from build123d import *

# Parameters (mm, degrees)
SKETCH_W      = 50.4
SKETCH_H      = 43.3
PAD_DEPTH     = 1.6
SKETCH001_R   = 1.65
HOLE_DEPTH    = 1.601
SKETCH002_W   = 10
SKETCH002_H   = 5.6
SKETCH002_W_2 = 5.6
SKETCH002_H_2 = 10
SKETCH002_W_3 = 5.7
SKETCH002_H_3 = 7.6
SKETCH002_W_4 = 7.6
SKETCH002_H_4 = 5.7
SKETCH002_H_5 = 9.8
PAD001_DEPTH  = 10.3


with BuildPart() as part:
    # Sketch → Pad (new body)
    with BuildSketch(Plane.XY):
        Rectangle(SKETCH_W, SKETCH_H)
    extrude(amount=PAD_DEPTH)

    # Sketch001 (on Face6 of Pad) → Hole (cut, through all)
    with BuildSketch(Plane.XY.offset(1.6)):
        with Locations((-22, 18.45)):
            Circle(SKETCH001_R)
        with Locations((22, 18.45)):
            Circle(SKETCH001_R)
        with Locations((-22, -18.45)):
            Circle(SKETCH001_R)
        with Locations((22, -18.45)):
            Circle(SKETCH001_R)
    extrude(amount=-HOLE_DEPTH, mode=Mode.SUBTRACT)

    # Sketch002 (on Face5 of Hole) → Pad001 (join)
    with BuildSketch(Plane.XY.offset(1.6)):
        with Locations((9.4, -17.35)):
            Rectangle(SKETCH002_W, SKETCH002_H)
        with Locations((-3.6, -17.35)):
            Rectangle(SKETCH002_W, SKETCH002_H)
        with Locations((-15.2, -14.25)):
            Rectangle(SKETCH002_W_2, SKETCH002_H_2)
        with Locations((-16.25, 9.05)):
            Rectangle(SKETCH002_W_3, SKETCH002_H_3)
        with Locations((5.2, 17.7)):
            Rectangle(SKETCH002_W_4, SKETCH002_H_4)
        with Locations((17.8, -8.15)):
            Rectangle(SKETCH002_W_4, SKETCH002_H_5)
    extrude(amount=PAD001_DEPTH)


solid = part.part
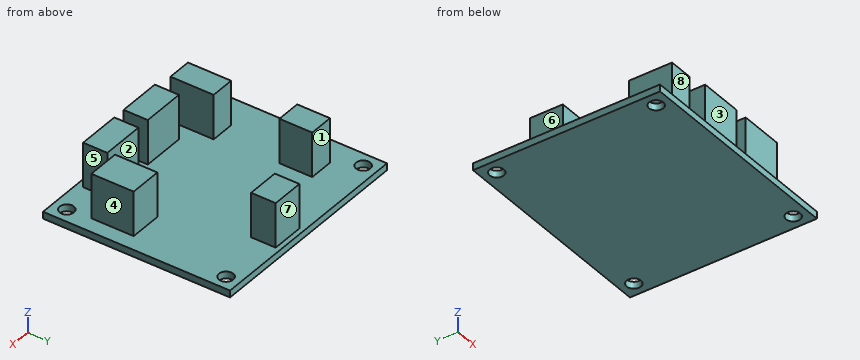
Work out the finished part from the listing and answer in its coordinate system (mm). Face numbers are marked on the shaded views. A direction names the side the tool comes from. Give positions to 0.01 mm unless a question says otherwise; leave off trailing zeros. Order: outer loops, then holes, each group sorted by start corner. A loop starts at its lowest first (then second) coordinate and runs counter-clockwise, first axis right, second up. Notation, with made-up numbers: M -5,-3.5 L 36,-3.5 A3 ccw 36,0.5 Z; hole C -13.5,-13 d6. An arc over 180 degrees is marked long. Return JSON: item names as keys, results as strings.
Q1. Find the intervals of material crossed by line 1 along X through (y, z) = (-15.5, 9); line 2 along Y through (x, z) = (-22, 0.75); line 3 along Z through (x, y) = (7, -6.5), in increasing order. Write a range as [from, to].
Answer below:
{"line 1": "x = [-18, -12.4], [-8.6, 1.4], [4.4, 14.4]", "line 2": "y = [-21.65, -20.1], [-16.8, 16.8], [20.1, 21.65]", "line 3": "z = [0, 1.6]"}
Q2. Find section B-B, the plane z = 4.5. Write down the section's boundary in (x, y).
Answer below:
{"outline": "M -19.1,5.25 L -13.4,5.25 L -13.4,12.85 L -19.1,12.85 Z; M -18,-19.25 L -12.4,-19.25 L -12.4,-9.25 L -18,-9.25 Z; M -8.6,-20.15 L 1.4,-20.15 L 1.4,-14.55 L -8.6,-14.55 Z; M 1.4,14.85 L 9,14.85 L 9,20.55 L 1.4,20.55 Z; M 4.4,-20.15 L 14.4,-20.15 L 14.4,-14.55 L 4.4,-14.55 Z; M 14,-13.05 L 21.6,-13.05 L 21.6,-3.25 L 14,-3.25 Z"}
Q3. Find section D-D, the plane x = -22. Write down the section's boundary in (y, z).
Answer below:
{"outline": "M -21.65,0 L -20.1,0 L -20.1,1.6 L -21.65,1.6 Z; M -16.8,0 L 16.8,0 L 16.8,1.6 L -16.8,1.6 Z; M 20.1,0 L 21.65,0 L 21.65,1.6 L 20.1,1.6 Z"}
Q4. Which of the six approach directions +Z, -Z, +X, -X, +Y, -Y give full straight-line access (tool end or side, diameter ignored) to the marked faces 5, 6, 7 and 8?
Answer below:
{"face 5": "+Z, +X, -Y", "face 6": "+Z, -X, +Y, -Y", "face 7": "+Z, +X, -X, +Y", "face 8": "+Z, -X, -Y"}
Q5. Find section A-A, the plane y = 18.45. Write down the section's boundary in (x, z).
Answer below:
{"outline": "M -25.2,0 L -23.65,0 L -23.65,1.6 L -25.2,1.6 Z; M -20.35,0 L 20.35,0 L 20.35,1.6 L 9,1.6 L 9,11.9 L 1.4,11.9 L 1.4,1.6 L -20.35,1.6 Z; M 23.65,0 L 25.2,0 L 25.2,1.6 L 23.65,1.6 Z"}
Q6. The mould has two halves that part along Y. Classify the marked faces 1, 2, 3 and 4: pulls with the +Y half, pulls with the -Y half, needs draft (parallel to the pull), parting line crosses it, or undercut.
Answer below:
{"face 1": "pulls with the +Y half", "face 2": "undercut", "face 3": "pulls with the -Y half", "face 4": "needs draft"}
Q7. Find section C-C, the plane x = 5. Write down the section's boundary in (y, z), and give its area (3 significant figures).
Answer below:
{"outline": "M -21.65,0 L 21.65,0 L 21.65,1.6 L 20.55,1.6 L 20.55,11.9 L 14.85,11.9 L 14.85,1.6 L -14.55,1.6 L -14.55,11.9 L -20.15,11.9 L -20.15,1.6 L -21.65,1.6 Z", "area": "186 mm^2"}
Q8. Each of these flat-tipped pins is pushed along its axis until it touches: pin 1 (3 mm diameter, centred on x = -4, z = 9, fed in from +Y); pin 2 (4.5 mm diameter, centred on x = -15.5, z = 8, fed in from -Y); pin 3 (3 mm diameter, centred on x = -3, z = 5.5, fed in from -Y). Where does it stop, or does it pass through?
Answer below:
{"pin 1": "stops at y = -14.55", "pin 2": "stops at y = -19.25", "pin 3": "stops at y = -20.15"}
